Input: part model. Units: mm. Frame: model coordinates. Face numbers are marked on the shaded views. A direction names the side the tool comes from. Round coordinates to 2 decimals unless told otherwise and drop trailing zeros. Order: outer loops, then holes, each group sorted by start corner. A loop starts at its lowest first (then second) coordinate and runs counter-clockwise, first axis right, second up. Notation, with made-up numbers: (84.25, 49) -> (126.25, 49) arc R33 cw to (126.25, 87) -> close; hole circle Ø9 at (77, -8). An arc over 180 degrees is marked (long way). Use a Markdown table: item, result.
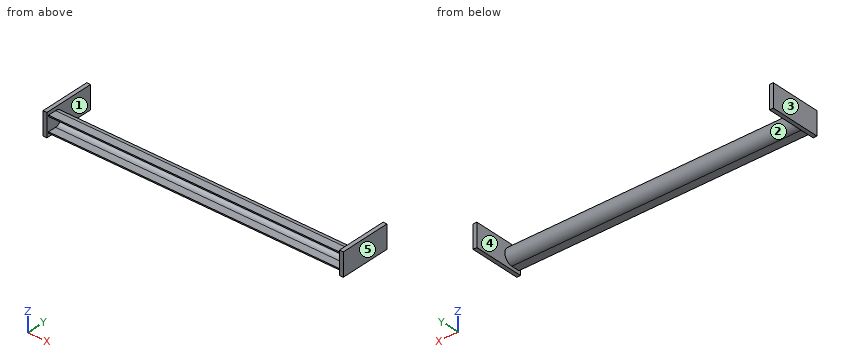
from build123d import *

# Parameters (mm, degrees)
SKETCH1_W           = 76.2
SKETCH1_H           = 168.275
BOSS_EXTRUDE1_DEPTH = 12.7
BOSS_EXTRUDE2_DEPTH = 965.2
SKETCH3_W           = 76.2
SKETCH3_H           = 168.275
BOSS_EXTRUDE3_DEPTH = 12.7


with BuildPart() as part:
    # Sketch1 → Boss-Extrude1 (new body)
    with BuildSketch(Plane(origin=(0, 0, 0), x_dir=(0, 0, -1), z_dir=(1, 0, 0))):
        Rectangle(SKETCH1_W, SKETCH1_H)
    extrude(amount=BOSS_EXTRUDE1_DEPTH)

    # Sketch2 → Boss-Extrude2 (add)
    with BuildSketch(Plane.ZY):
        with BuildLine():
            Line((-26.9875, -77.7875), (-26.9875, -50.8))
            ThreePointArc((-26.9875, -50.8), (0, -23.8125), (26.9875, -50.8))
            Line((26.9875, -50.8), (26.9875, -77.7875))
            Line((26.9875, -77.7875), (22.9235, -77.7875))
            Line((22.9235, -77.7875), (22.9235, -50.8))
            ThreePointArc((22.9235, -50.8), (0, -27.8765), (-22.9235, -50.8))
            Line((-22.9235, -50.8), (-22.9235, -77.7875))
            Line((-22.9235, -77.7875), (-26.9875, -77.7875))
        make_face()
    extrude(amount=BOSS_EXTRUDE2_DEPTH)

    # Sketch3 → Boss-Extrude3 (add)
    with BuildSketch(Plane.ZY.offset(965.2)):
        Rectangle(SKETCH3_W, SKETCH3_H)
    extrude(amount=BOSS_EXTRUDE3_DEPTH)


solid = part.part
1) Cut plane A-A on y = 64. Return loops of the section in (x, z), and give its area (3 significant figures).
Results found:
| item | result |
|---|---|
| outline | (-977.9, -38.1) -> (-965.2, -38.1) -> (-965.2, 38.1) -> (-977.9, 38.1) -> close; (0, -38.1) -> (12.7, -38.1) -> (12.7, 38.1) -> (0, 38.1) -> close |
| area | 1,940 mm² |
2) Set-up query: the marked faces 1 and 2. Return all of +Z, -Z, +X, -X, +Y, -Y with unobstructed straight access to the full face (end or side cutting, diameter ignored); none if empty.
Results found:
| item | result |
|---|---|
| face 1 | none |
| face 2 | +Y |
3) Line query: L1, parallel to X at y = 50, z = 28.5; L2, parallel to Z at x = -404, y = -58; L3, parallel to Y at x = -623.5, z = -3. Output: solid intervals per line, ascending. Write a range as [from, to].
Results found:
| item | result |
|---|---|
| L1 | x = [-977.9, -965.2], [0, 12.7] |
| L2 | z = [-26.99, -22.92], [22.92, 26.99] |
| L3 | y = [-28.07, -23.98] |
4) Pin query (flat end, axial travel): pin 1 Ø13.5 at (x, y) = (-683.5, -61) entering from -Z; pin 2 Ø13.5 at (x, y) = (-467.5, -64) entering from +Z; pin 3 Ø2 at (x, z) = (-663.5, 25.5) entering from -Y. Return the tip coordinate at first contact, or that it passes through.
Results found:
| item | result |
|---|---|
| pin 1 | stops at z = -26.99 |
| pin 2 | stops at z = 26.99 |
| pin 3 | stops at y = -77.79 |
5) Cut plane C-C on x = -515. Return loops of the section in (y, z) (1 decimal), and give its area (3 significant figures).
Results found:
| item | result |
|---|---|
| outline | (-77.8, -27) -> (-50.8, -27) arc R27 ccw to (-50.8, 27) -> (-77.8, 27) -> (-77.8, 22.9) -> (-50.8, 22.9) arc R22.9 cw to (-50.8, -22.9) -> (-77.8, -22.9) -> close |
| area | 538 mm² |
6) Pull-direction query (X, two-part tool) for the marked faces 3, 4 and 5; classes: +X half, -X half, draft (parallel to the pull), parting line (faces both ways), or undercut.
Results found:
| item | result |
|---|---|
| face 3 | -X half |
| face 4 | undercut |
| face 5 | +X half |
7) Cut plane B-B on z = 0. Return loops of the section in (x, y), and give its area (3 significant figures).
Results found:
| item | result |
|---|---|
| outline | (-977.9, -84.14) -> (-965.2, -84.14) -> (-965.2, -27.88) -> (0, -27.88) -> (0, -84.14) -> (12.7, -84.14) -> (12.7, 84.14) -> (0, 84.14) -> (0, -23.81) -> (-965.2, -23.81) -> (-965.2, 84.14) -> (-977.9, 84.14) -> close |
| area | 8,200 mm² |
